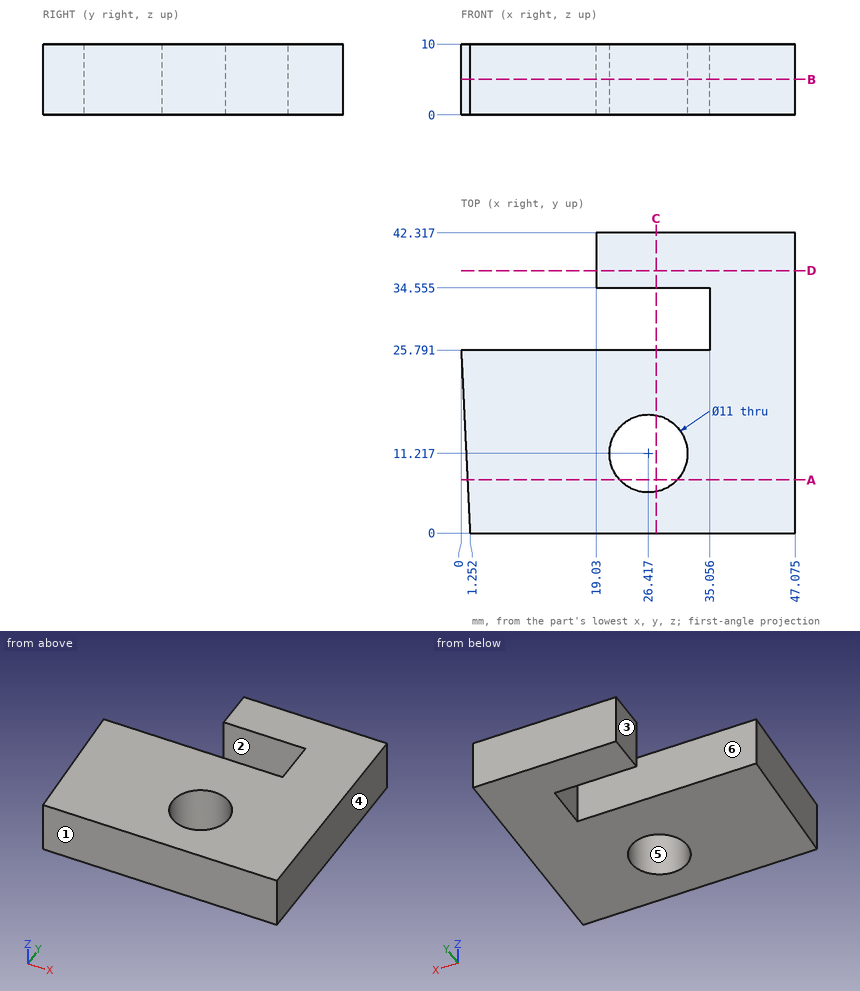
Part print with two shaded views. Sizes in mm from the minimum x, y, z corner. A direction names the side the tool comes from. Round coordinates to 2 decimals unless told otherwise and drop trailing zeros. Order: outer loops, then holes, each group sorted by start corner. A loop starts at its lowest first (then second) coordinate and runs counter-clockwise, first axis right, second up.
(1) Band-saw the part on B-B (z = 5). List the corners of the cut face in (x, y) (1 decimal), then the cut area to 3 significant figures.
(2) Drill centre lines: line 1 (Y direction, x = 34, z = 4) (1 decimal); line 2 (X direction, y = 27.5, z = 5.5) (1 decimal); line 3 (Y direction, x = 2, z = 5.5). Where is each one in solid material? Low to high.
(3) Band-saw the part on C-C (x = 27.5). List the corners of the cut face in (y, z) (1 decimal), then the cut area to 3 significant figures.
(4) Pin check, flat tips, straight feed: pin 1 (1 mm diameter, centred on x = 16, z = 5, fed in from +Y); pin 2 (3 mm diameter, centred on y = 23, z = 7.5, fed in from -X); pin 3 (10 mm diameter, centred on x = 26.42, y = 11.22, fed in from +Z); pin 4 (6 mm diameter, centred on y = 40, z = 3, fed in from -X). Stop position of each tip, or through.
(5) Band-saw the part on A-A (y = 7.5). List the corners of the cut face in (x, z) (1 decimal).
(6) 3-axis set-ups, long thin cutter, end or side, ignore diameter. For the marked faces 1 and 2: which of +Z, -Z, +X, -X, +Y, -Y reach the whole face in a straight line?
(7) Band-saw the part on D-D (y = 37). List the corners of the cut face in (x, z) (1 decimal), then the cut area to 3 significant figures.
(8) Pull direction X, two halves, no side cores. Call the marked faces 3, 4, 5 and 6: released by +X, released by -X, zero draft, split by the parting line, or undercut.
Verdict:
1. outline: (0, 25.8) - (1.3, 0) - (47.1, 0) - (47.1, 42.3) - (19, 42.3) - (19, 34.6) - (35.1, 34.6) - (35.1, 25.8) - close; hole circle Ø11 at (26.4, 11.2)
1. area: 1,430 mm2
2. line 1: y = 0 to 25.8, 34.6 to 42.3
2. line 2: x = 35.1 to 47.1
2. line 3: y = 0 to 25.79
3. outline: (0, 0) - (5.8, 0) - (5.8, 10) - (0, 10) - close; (16.6, 0) - (25.8, 0) - (25.8, 10) - (16.6, 10) - close; (34.6, 0) - (42.3, 0) - (42.3, 10) - (34.6, 10) - close
3. area: 228 mm2
4. pin 1: stops at y = 25.79
4. pin 2: stops at x = 0.06
4. pin 3: passes through
4. pin 4: stops at x = 19.03
5. outline: (0.9, 0) - (22.4, 0) - (22.4, 10) - (0.9, 10) - close; (30.5, 0) - (47.1, 0) - (47.1, 10) - (30.5, 10) - close
6. face 1: +Z, -Z, +X, -X, -Y
6. face 2: +Z, -Z, -X
7. outline: (19, 0) - (47.1, 0) - (47.1, 10) - (19, 10) - close
7. area: 280 mm2
8. face 3: released by -X
8. face 4: released by +X
8. face 5: undercut
8. face 6: zero draft
